Drawing for the job (mm, zero at the part's lowest x, y, z). A direction names the side the tool comes from. Give positions to 0.01 mm unless a question says otherwise; leave off trailing zeros. Order: outer loops, then holes, each group sorted by start corner. A loop starts at its lowest first (then second) coordinate and runs counter-clockwise, first axis right, second up. Notation, with made-up numbers: (2, -30.75) - (47, -30.75) arc R13 ccw to (47, -14.75) - close; hole circle Ø2 at (-11.75, 82). An arc over 180 degrees is marked (long way). Use a Markdown table: item, result.
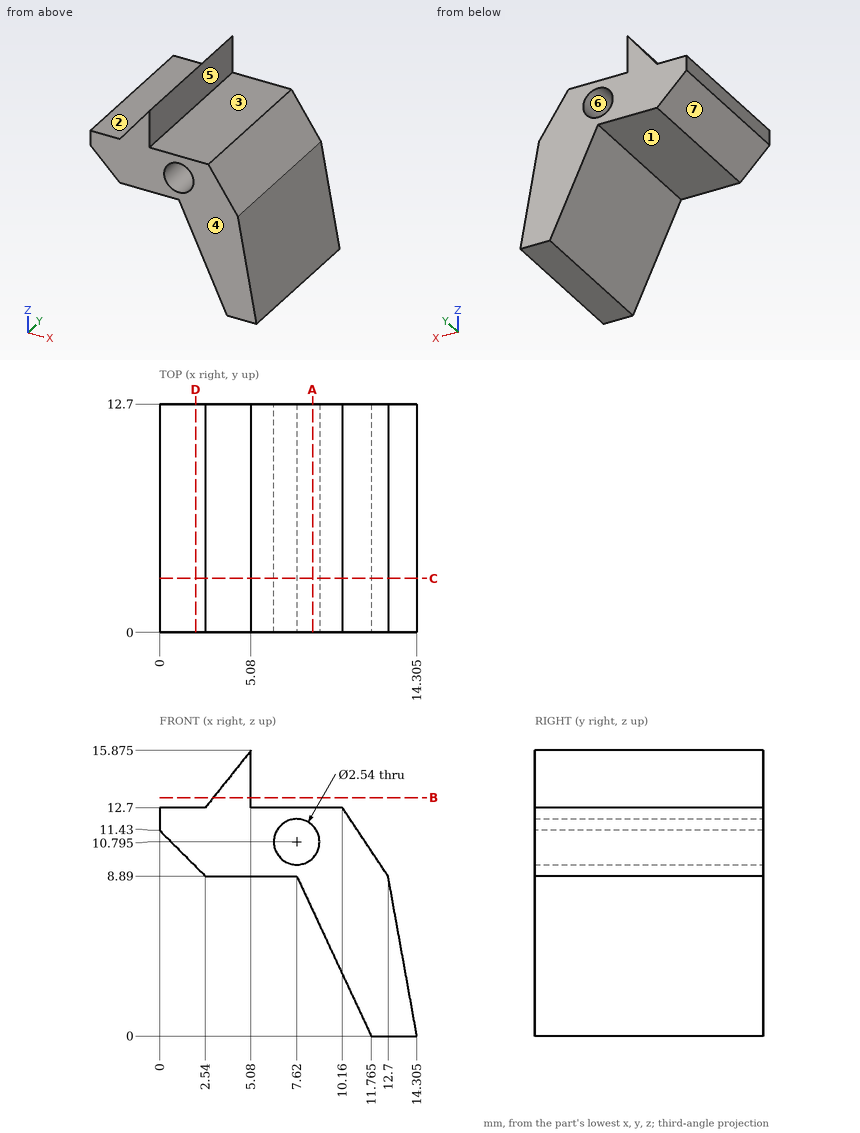
1) Slice it at B-B (z = 13.25). Write the cut outline in (x, y).
Computed:
| item | result |
|---|---|
| outline | (2.98, 0) - (5.08, 0) - (5.08, 12.7) - (2.98, 12.7) - close |
2) Two-plate mould, pull along X, no slides. Class the marked faces 4, 5, 6 and 7: +X half, -X half, draft (parallel to the pull), parting line (faces both ways), or undercut.
Computed:
| item | result |
|---|---|
| face 4 | draft |
| face 5 | +X half |
| face 6 | undercut |
| face 7 | -X half |
3) Slice it at A-A (x = 8.5). Write the cut outline in (y, z).
Computed:
| item | result |
|---|---|
| outline | (0, 7) - (12.7, 7) - (12.7, 9.88) - (0, 9.88) - close; (0, 11.71) - (12.7, 11.71) - (12.7, 12.7) - (0, 12.7) - close |
4) Wall check: line 1 (X direction, y = 3.5, z = 10.75); line 2 (X direction, y = 2.75, z = 11.25) (1 decimal); line 3 (X direction, y = 9.75, z = 13.5). Give the ranges that are in metal, low to high. Write a range as from..to.
Computed:
| item | result |
|---|---|
| line 1 | x = 0.68..6.35, 8.89..11.46 |
| line 2 | x = 0.2..6.4, 8.8..11.1 |
| line 3 | x = 3.18..5.08 |
5) Tool access for the marked faces 1, 2 and 3: list every direction of +Z, -Z, +X, -X, +Y, -Y with a clear straight run to the whole face (end or side of a thin tool).
Computed:
| item | result |
|---|---|
| face 1 | -Z, -X, +Y, -Y |
| face 2 | +Z, -X, +Y, -Y |
| face 3 | +Z, +X, +Y, -Y |
6) Slice it at C-C (y = 3). Write the cut outline in (x, z) (1 decimal).
Computed:
| item | result |
|---|---|
| outline | (0, 11.4) - (2.5, 8.9) - (7.6, 8.9) - (11.8, 0) - (14.3, 0) - (12.7, 8.9) - (10.2, 12.7) - (5.1, 12.7) - (5.1, 15.9) - (2.5, 12.7) - (0, 12.7) - close; hole circle Ø2.5 at (7.6, 10.8) |
7) Slice it at D-D (x = 2). Write the cut outline in (y, z).
Computed:
| item | result |
|---|---|
| outline | (0, 9.43) - (12.7, 9.43) - (12.7, 12.7) - (0, 12.7) - close |
8) Pin check, flat tips, straight feed: P1, Ø0.8, axis at x = 1, y = 4.5, coming from the +Z side; P2, Ø4, axis at x = 5.5, y = 5, coming from the -Z side; P3, Ø5, axis at y = 6.5, z = 10.5, coming from the -X side; P4, Ø3, axis at x = 12, y = 4, coming from the +Z side. Stop position of each tip, or through.
Computed:
| item | result |
|---|---|
| P1 | stops at z = 12.7 |
| P2 | stops at z = 8.89 |
| P3 | stops at x = 0 |
| P4 | stops at z = 12.19 |
